Geometry: final body of the model. Coordinates: model frame, mm. Face numbers are marked on the shaded views. A direction names the side the tool comes from. Give positions to 0.01 mm unless a question says otherwise; leave off trailing zeros. Loops run counter-clockwise (first coordinate to the right, second up) from the corner with the lowest first, then second, coordinate; pieces in that order, holes last. Notation, with made-up numbers: M 0,28 L 26,28 A25 ccw 26,50 Z; hole C 69,-9.75 d6. An arc over 180 degrees is marked long. One line per question, with ' | ' between items. Start each with the question number.
from build123d import *

# Parameters (mm, degrees)
SKETCH1_W            = 70
SKETCH1_H            = 60
BOSS_EXTRUDE2_DEPTH  = 5
SKETCH15_W           = 29
SKETCH15_H           = 9
BOSS_EXTRUDE13_DEPTH = 20
SKETCH16_R           = 5.5
CUT_EXTRUDE3_DEPTH   = 54.058929503
FILLET1_R            = 2


with BuildPart() as part:
    # Sketch1 → Boss-Extrude2 (new body)
    with BuildSketch(Plane(origin=(0, 0, 0), x_dir=(1, 0, 0), z_dir=(0, 1, 0))):
        Rectangle(SKETCH1_W, SKETCH1_H)
    extrude(amount=BOSS_EXTRUDE2_DEPTH)

    # Sketch15 → Boss-Extrude13 (add)
    with BuildSketch(Plane(origin=(0, 0, 0), x_dir=(-1, 0, 0), z_dir=(0, 1, 0))):
        Rectangle(SKETCH15_W, SKETCH15_H)
    extrude(amount=-BOSS_EXTRUDE13_DEPTH)

    # Sketch16 → Cut-Extrude3 (cut, through all)
    with BuildSketch(Plane.XY.offset(4.5)):
        with Locations((0, -12)):
            Circle(SKETCH16_R)
    extrude(amount=-CUT_EXTRUDE3_DEPTH, mode=Mode.SUBTRACT)

    # Fillet1
    fillet1_edges = [part.edges().sort_by_distance(p)[0] for p in [
        (-14.5, -20, 0),
        (-14.5, -10, 4.5),
        (0, -20, -4.5),
        (-14.5, -10, -4.5),
        (14.5, -20, 0),
        (14.5, -10, -4.5),
        (0, -20, 4.5),
        (14.5, -10, 4.5),
        (-14.5, 0, 0),
        (0, 0, 4.5),
        (14.5, 0, 0),
        (0, 0, -4.5),
        (35, 2.5, 30),
        (-35, 2.5, 30),
        (-35, 2.5, -30),
        (35, 2.5, -30),
    ]]
    fillet(fillet1_edges, radius=FILLET1_R)


solid = part.part
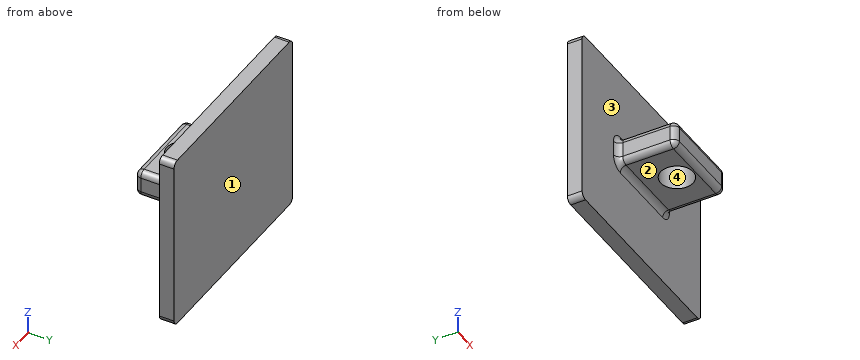
Q1. Section B-B, the plane y = -12. Output: boundary loops of the cut face in (x, z), plus the area to 3 significant figures.
Q2. Set-up query: the marked faces 1 and 2. Return all of +Z, -Z, +X, -X, +Y, -Y with unobstructed straight access to the full face (end or side cutting, diameter ignored); none if empty.
Q3. Contact query for flat-ended pins moving along their axis: pin 1 (1 mm diameter, centred on x = -9, z = 11, fed in from -Y); pin 2 (12 mm diameter, centred on x = -18, y = -1.5, fed in from -Z); pin 3 (5 mm diameter, centred on x = -6, y = -10.5, fed in from +Z); pin 4 (8 mm diameter, centred on x = -6, y = -9.5, fed in from -Z). Output: stop coordinate, or through.
Q4. Material intervals for L1, parallel to Y at x = 0, z = 0; L2, parallel to Z at x = -8, y = -8.25; L3, parallel to Y at x = -10, z = -8.5, sorted ascending.
Q5. Section A-A, the plane x = 0. Output: boundary loops of the cut face in (y, z).
Q6. Section C-C, the plane z = -1. Output: boundary loops of the cut face in (x, y).
Q7. Section D-D, the plane y = -5. Output: boundary loops of the cut face in (x, z).
Q8. Draft query along X for the marked faces 3 and 4. Return one class per face: released by +X, released by -X, zero draft, split by the parting line, or undercut.
Model answer:
1) outline: M -14.5,-2.5 A2 ccw -12.5,-4.5 L -5.5,-4.5 L -5.5,4.5 L -12.5,4.5 A2 ccw -14.5,2.5 Z; M 5.5,-4.5 L 12.5,-4.5 A2 ccw 14.5,-2.5 L 14.5,2.5 A2 ccw 12.5,4.5 L 5.5,4.5 Z | area: 159 mm^2
2) face 1: +Z, -Z, +X, -X, +Y | face 2: -Z, +X, -X, -Y
3) pin 1: stops at y = 0 | pin 2: stops at z = -30 | pin 3: stops at z = 4.5 | pin 4: stops at z = -4.5
4) L1: y = -20 to -17.5, -6.5 to 5 | L2: z = -4.5 to 4.5 | L3: y = 0 to 5
5) outline: M -20,-2.5 A2 ccw -18,-4.5 L -17.5,-4.5 L -17.5,4.5 L -18,4.5 A2 ccw -20,2.5 Z; M -6.5,-4.5 L -2,-4.5 A2 cw 0,-6.5 L 0,-30 L 5,-30 L 5,30 L 0,30 L 0,6.5 A2 cw -2,4.5 L -6.5,4.5 Z
6) outline: M -35,0 L -16.5,0 A2 cw -14.5,-2 L -14.5,-18 A2 ccw -12.5,-20 L 12.5,-20 A2 ccw 14.5,-18 L 14.5,-2 A2 cw 16.5,0 L 35,0 L 35,5 L -35,5 Z; hole C 0,-12 d11
7) outline: M -14.5,-2.5 A2 ccw -12.5,-4.5 L 12.5,-4.5 A2 ccw 14.5,-2.5 L 14.5,2.5 A2 ccw 12.5,4.5 L -12.5,4.5 A2 ccw -14.5,2.5 Z
8) face 3: zero draft | face 4: undercut
